from build123d import *

# Parameters (mm, degrees)
F0_R     = 2.25
F1_DEPTH = 0.2
F2_DEPTH = 1.2


with BuildPart() as f1:
    # F0 (on Top) → F1 (new body)
    with BuildSketch(Plane.XY):
        with BuildLine():
            Line((0.7, -5.554778), (0.7, -4.445222))
            ThreePointArc((0.7, -4.445222), (0, -4.5), (-0.7, -4.445222))
            Line((-0.7, -4.445222), (-0.7, -5.554778))
            ThreePointArc((-0.7, -5.554778), (0, -5.5), (0.7, -5.554778))
        make_face()
        with BuildLine():
            ThreePointArc((4.445222, 0.7), (4.486285, 0.35107), (4.5, 0))
            ThreePointArc((4.5, 0), (4.486285, -0.35107), (4.445222, -0.7))
            Line((4.445222, -0.7), (5.554778, -0.7))
            ThreePointArc((5.554778, -0.7), (5.5, 0), (5.554778, 0.7))
            Line((5.554778, 0.7), (4.445222, 0.7))
        make_face()
        with BuildLine():
            Line((5.554778, -9.3), (4.445222, -9.3))
            ThreePointArc((4.445222, -9.3), (4.486285, -9.64893), (4.5, -10))
            ThreePointArc((4.5, -10), (4.486285, -10.35107), (4.445222, -10.7))
            Line((4.445222, -10.7), (5.554778, -10.7))
            ThreePointArc((5.554778, -10.7), (5.5, -10), (5.554778, -9.3))
        make_face()
        with BuildLine():
            Line((15.554778, 0.7), (14.445222, 0.7))
            ThreePointArc((14.445222, 0.7), (14.486285, 0.35107), (14.5, 0))
            ThreePointArc((14.5, 0), (14.486285, -0.35107), (14.445222, -0.7))
            Line((14.445222, -0.7), (15.554778, -0.7))
            ThreePointArc((15.554778, -0.7), (15.5, 0), (15.554778, 0.7))
        make_face()
        with BuildLine():
            Line((15.554778, -9.3), (14.445222, -9.3))
            ThreePointArc((14.445222, -9.3), (14.486285, -9.64893), (14.5, -10))
            ThreePointArc((14.5, -10), (14.486285, -10.35107), (14.445222, -10.7))
            Line((14.445222, -10.7), (15.554778, -10.7))
            ThreePointArc((15.554778, -10.7), (15.5, -10), (15.554778, -9.3))
        make_face()
        with BuildLine():
            ThreePointArc((20.7, -4.445222), (20, -4.5), (19.3, -4.445222))
            Line((19.3, -4.445222), (19.3, -5.554778))
            ThreePointArc((19.3, -5.554778), (20, -5.5), (20.7, -5.554778))
            Line((20.7, -5.554778), (20.7, -4.445222))
        make_face()
        with BuildLine():
            ThreePointArc((4.445222, -9.3), (3.181981, -6.818019), (0.7, -5.554778))
            ThreePointArc((0.7, -5.554778), (0, -5.5), (-0.7, -5.554778))
            ThreePointArc((-0.7, -5.554778), (-4.5, -10), (-0.7, -14.445222))
            ThreePointArc((-0.7, -14.445222), (0, -14.5), (0.7, -14.445222))
            ThreePointArc((0.7, -14.445222), (3.181981, -13.181981), (4.445222, -10.7))
            ThreePointArc((4.445222, -10.7), (4.486285, -10.35107), (4.5, -10))
            ThreePointArc((4.5, -10), (4.486285, -9.64893), (4.445222, -9.3))
        make_face()
        with Locations((0, -10)):
            Circle(F0_R, mode=Mode.SUBTRACT)
        with BuildLine():
            ThreePointArc((24.445222, 0.7), (20, 4.5), (15.554778, 0.7))
            ThreePointArc((15.554778, 0.7), (15.5, 0), (15.554778, -0.7))
            ThreePointArc((15.554778, -0.7), (16.818019, -3.181981), (19.3, -4.445222))
            ThreePointArc((19.3, -4.445222), (20, -4.5), (20.7, -4.445222))
            ThreePointArc((20.7, -4.445222), (23.181981, -3.181981), (24.445222, -0.7))
            ThreePointArc((24.445222, -0.7), (24.486285, -0.35107), (24.5, 0))
            ThreePointArc((24.5, 0), (24.486285, 0.35107), (24.445222, 0.7))
        make_face()
        with Locations((20, 0)):
            Circle(F0_R, mode=Mode.SUBTRACT)
        with BuildLine():
            ThreePointArc((20.7, -5.554778), (20, -5.5), (19.3, -5.554778))
            ThreePointArc((19.3, -5.554778), (16.818019, -6.818019), (15.554778, -9.3))
            ThreePointArc((15.554778, -9.3), (15.5, -10), (15.554778, -10.7))
            ThreePointArc((15.554778, -10.7), (16.818019, -13.181981), (19.3, -14.445222))
            ThreePointArc((19.3, -14.445222), (20, -14.5), (20.7, -14.445222))
            ThreePointArc((20.7, -14.445222), (23.181981, -13.181981), (24.445222, -10.7))
            ThreePointArc((24.445222, -10.7), (24.486285, -10.35107), (24.5, -10))
            ThreePointArc((24.5, -10), (24.486285, -9.64893), (24.445222, -9.3))
            ThreePointArc((24.445222, -9.3), (23.181981, -6.818019), (20.7, -5.554778))
        make_face()
        with Locations((20, -10)):
            Circle(F0_R, mode=Mode.SUBTRACT)
        with BuildLine():
            ThreePointArc((14.445222, 0.7), (10, 4.5), (5.554778, 0.7))
            ThreePointArc((5.554778, 0.7), (5.5, 0), (5.554778, -0.7))
            ThreePointArc((5.554778, -0.7), (6.818019, -3.181981), (9.3, -4.445222))
            ThreePointArc((9.3, -4.445222), (10, -4.5), (10.7, -4.445222))
            ThreePointArc((10.7, -4.445222), (13.181981, -3.181981), (14.445222, -0.7))
            ThreePointArc((14.445222, -0.7), (14.486285, -0.35107), (14.5, 0))
            ThreePointArc((14.5, 0), (14.486285, 0.35107), (14.445222, 0.7))
        make_face()
        with Locations((10, 0)):
            Circle(F0_R, mode=Mode.SUBTRACT)
        with BuildLine():
            ThreePointArc((10.7, -5.554778), (10, -5.5), (9.3, -5.554778))
            ThreePointArc((9.3, -5.554778), (6.818019, -6.818019), (5.554778, -9.3))
            ThreePointArc((5.554778, -9.3), (5.5, -10), (5.554778, -10.7))
            ThreePointArc((5.554778, -10.7), (6.818019, -13.181981), (9.3, -14.445222))
            ThreePointArc((9.3, -14.445222), (10, -14.5), (10.7, -14.445222))
            ThreePointArc((10.7, -14.445222), (13.181981, -13.181981), (14.445222, -10.7))
            ThreePointArc((14.445222, -10.7), (14.486285, -10.35107), (14.5, -10))
            ThreePointArc((14.5, -10), (14.486285, -9.64893), (14.445222, -9.3))
            ThreePointArc((14.445222, -9.3), (13.181981, -6.818019), (10.7, -5.554778))
        make_face()
        with Locations((10, -10)):
            Circle(F0_R, mode=Mode.SUBTRACT)
        with BuildLine():
            ThreePointArc((4.445222, -0.7), (4.486285, -0.35107), (4.5, 0))
            ThreePointArc((4.5, 0), (4.486285, 0.35107), (4.445222, 0.7))
            ThreePointArc((4.445222, 0.7), (0, 4.5), (-4.445222, 0.7))
            ThreePointArc((-4.445222, 0.7), (-4.5, 0), (-4.445222, -0.7))
            ThreePointArc((-4.445222, -0.7), (-3.181981, -3.181981), (-0.7, -4.445222))
            ThreePointArc((-0.7, -4.445222), (0, -4.5), (0.7, -4.445222))
            ThreePointArc((0.7, -4.445222), (3.181981, -3.181981), (4.445222, -0.7))
        make_face()
        Circle(F0_R, mode=Mode.SUBTRACT)
        with BuildLine():
            ThreePointArc((10.7, -4.445222), (10, -4.5), (9.3, -4.445222))
            Line((9.3, -4.445222), (9.3, -5.554778))
            ThreePointArc((9.3, -5.554778), (10, -5.5), (10.7, -5.554778))
            Line((10.7, -5.554778), (10.7, -4.445222))
        make_face()
    extrude(amount=-F1_DEPTH)

    # F0 (on Top) → F2 (join)
    with BuildSketch(Plane.XY):
        with BuildLine():
            ThreePointArc((4.445222, -0.7), (4.486285, -0.35107), (4.5, 0))
            ThreePointArc((4.5, 0), (4.486285, 0.35107), (4.445222, 0.7))
            ThreePointArc((4.445222, 0.7), (0, 4.5), (-4.445222, 0.7))
            ThreePointArc((-4.445222, 0.7), (-4.5, 0), (-4.445222, -0.7))
            ThreePointArc((-4.445222, -0.7), (-3.181981, -3.181981), (-0.7, -4.445222))
            ThreePointArc((-0.7, -4.445222), (0, -4.5), (0.7, -4.445222))
            ThreePointArc((0.7, -4.445222), (3.181981, -3.181981), (4.445222, -0.7))
        make_face()
        Circle(F0_R, mode=Mode.SUBTRACT)
        with BuildLine():
            ThreePointArc((14.445222, 0.7), (10, 4.5), (5.554778, 0.7))
            ThreePointArc((5.554778, 0.7), (5.5, 0), (5.554778, -0.7))
            ThreePointArc((5.554778, -0.7), (6.818019, -3.181981), (9.3, -4.445222))
            ThreePointArc((9.3, -4.445222), (10, -4.5), (10.7, -4.445222))
            ThreePointArc((10.7, -4.445222), (13.181981, -3.181981), (14.445222, -0.7))
            ThreePointArc((14.445222, -0.7), (14.486285, -0.35107), (14.5, 0))
            ThreePointArc((14.5, 0), (14.486285, 0.35107), (14.445222, 0.7))
        make_face()
        with Locations((10, 0)):
            Circle(F0_R, mode=Mode.SUBTRACT)
        with BuildLine():
            ThreePointArc((24.445222, 0.7), (20, 4.5), (15.554778, 0.7))
            ThreePointArc((15.554778, 0.7), (15.5, 0), (15.554778, -0.7))
            ThreePointArc((15.554778, -0.7), (16.818019, -3.181981), (19.3, -4.445222))
            ThreePointArc((19.3, -4.445222), (20, -4.5), (20.7, -4.445222))
            ThreePointArc((20.7, -4.445222), (23.181981, -3.181981), (24.445222, -0.7))
            ThreePointArc((24.445222, -0.7), (24.486285, -0.35107), (24.5, 0))
            ThreePointArc((24.5, 0), (24.486285, 0.35107), (24.445222, 0.7))
        make_face()
        with Locations((20, 0)):
            Circle(F0_R, mode=Mode.SUBTRACT)
        with BuildLine():
            ThreePointArc((20.7, -5.554778), (20, -5.5), (19.3, -5.554778))
            ThreePointArc((19.3, -5.554778), (16.818019, -6.818019), (15.554778, -9.3))
            ThreePointArc((15.554778, -9.3), (15.5, -10), (15.554778, -10.7))
            ThreePointArc((15.554778, -10.7), (16.818019, -13.181981), (19.3, -14.445222))
            ThreePointArc((19.3, -14.445222), (20, -14.5), (20.7, -14.445222))
            ThreePointArc((20.7, -14.445222), (23.181981, -13.181981), (24.445222, -10.7))
            ThreePointArc((24.445222, -10.7), (24.486285, -10.35107), (24.5, -10))
            ThreePointArc((24.5, -10), (24.486285, -9.64893), (24.445222, -9.3))
            ThreePointArc((24.445222, -9.3), (23.181981, -6.818019), (20.7, -5.554778))
        make_face()
        with Locations((20, -10)):
            Circle(F0_R, mode=Mode.SUBTRACT)
        with BuildLine():
            ThreePointArc((10.7, -5.554778), (10, -5.5), (9.3, -5.554778))
            ThreePointArc((9.3, -5.554778), (6.818019, -6.818019), (5.554778, -9.3))
            ThreePointArc((5.554778, -9.3), (5.5, -10), (5.554778, -10.7))
            ThreePointArc((5.554778, -10.7), (6.818019, -13.181981), (9.3, -14.445222))
            ThreePointArc((9.3, -14.445222), (10, -14.5), (10.7, -14.445222))
            ThreePointArc((10.7, -14.445222), (13.181981, -13.181981), (14.445222, -10.7))
            ThreePointArc((14.445222, -10.7), (14.486285, -10.35107), (14.5, -10))
            ThreePointArc((14.5, -10), (14.486285, -9.64893), (14.445222, -9.3))
            ThreePointArc((14.445222, -9.3), (13.181981, -6.818019), (10.7, -5.554778))
        make_face()
        with Locations((10, -10)):
            Circle(F0_R, mode=Mode.SUBTRACT)
        with BuildLine():
            ThreePointArc((4.445222, -9.3), (3.181981, -6.818019), (0.7, -5.554778))
            ThreePointArc((0.7, -5.554778), (0, -5.5), (-0.7, -5.554778))
            ThreePointArc((-0.7, -5.554778), (-4.5, -10), (-0.7, -14.445222))
            ThreePointArc((-0.7, -14.445222), (0, -14.5), (0.7, -14.445222))
            ThreePointArc((0.7, -14.445222), (3.181981, -13.181981), (4.445222, -10.7))
            ThreePointArc((4.445222, -10.7), (4.486285, -10.35107), (4.5, -10))
            ThreePointArc((4.5, -10), (4.486285, -9.64893), (4.445222, -9.3))
        make_face()
        with Locations((0, -10)):
            Circle(F0_R, mode=Mode.SUBTRACT)
    extrude(amount=F2_DEPTH)


solid = f1.part
Input: part model. Units: mm. Frame: model coordinates. Give positions to 0.01 mm unless a question says otherwise; leave off trailing zeros. Order: outer loops, then holes, each group sorted by start corner. A loop starts at its lowest first (then second) coordinate and runs counter-clockwise, first axis right, second up. Notation, with made-up numbers: (-25.75, 86.5) - (9.25, 86.5) arc R35 cw to (9.25, 125.5) - close; hole circle Ø6 at (7.5, 58.5). An arc over 180 degrees is marked (long way). Answer as a JSON object with one key per item and string values. Group by question number.
Q1. Cut plane A-A, the plane x = 20. Output: boundary loops of the cut face in (y, z), then the cut area to 3 significant figures.
Q2. Line query: probe 1 along Y at (x, z) = (0, 0.35); probe 2 along X at (y, z) = (-10.25, 0.55); probe 3 along Y at (x, z) = (0, -0.05). Output: solid intervals per line, ascending.
Q3. Cut plane D-D, the plane y = -9. Output: boundary loops of the cut face in (x, z).
Q4. First-contact query: pin 1 Ø4 at (x, y) = (20, 0) entering from +Z; pin 2 Ø0.9 at (x, y) = (20, -5) entering from +Z. Flat tips, straight axial feed; report the tip coordinate or a pass-through.
Q5. Cut plane B-B, the plane z = 0.8. Count the separate pieces of the cut face and the enclosed holes in it, then the cut area to 3 significant figures.
Q6. Mould query, pull axis X, two halves, no side actions, for faces 1 (the face through (-4.5, -9.9, 0.5)), 2 (the face through (10.1, 4.5, 0.5)), 3 (the face through (2, -2, 1.2)). Classes: pulls with the +X half, pulls with the -X half, needs draft (parallel to the pull), parting line crosses it, or undercut.
Q7. Cut plane C-C, the plane y = -6.5. Output: boundary loops of the cut face in (x, z), then the cut area to 3 significant figures.
Results:
{
 "1": {"outline": "(-14.5, -0.2) - (-12.25, -0.2) - (-12.25, 1.2) - (-14.5, 1.2) - close; (-7.75, -0.2) - (-2.25, -0.2) - (-2.25, 1.2) - (-4.5, 1.2) - (-4.5, 0) - (-5.5, 0) - (-5.5, 1.2) - (-7.75, 1.2) - close; (2.25, -0.2) - (4.5, -0.2) - (4.5, 1.2) - (2.25, 1.2) - close", "area": "12.8 mm^2"},
 "2": {"probe 1": "-14.5 to -12.25, -7.75 to -5.5, -4.5 to -2.25, 2.25 to 4.5", "probe 2": "-4.49 to -2.24, 2.24 to 4.49, 5.51 to 7.76, 12.24 to 14.49, 15.51 to 17.76, 22.24 to 24.49", "probe 3": "-14.5 to -12.25, -7.75 to -2.25, 2.25 to 4.5"},
 "3": {"outline": "(-4.39, -0.2) - (-2.02, -0.2) - (-2.02, 1.2) - (-4.39, 1.2) - close; (2.02, -0.2) - (4.39, -0.2) - (4.39, 1.2) - (2.02, 1.2) - close; (5.61, -0.2) - (7.98, -0.2) - (7.98, 1.2) - (5.61, 1.2) - close; (12.02, -0.2) - (14.39, -0.2) - (14.39, 1.2) - (12.02, 1.2) - close; (15.61, -0.2) - (17.98, -0.2) - (17.98, 1.2) - (15.61, 1.2) - close; (22.02, -0.2) - (24.39, -0.2) - (24.39, 1.2) - (22.02, 1.2) - close"},
 "4": {"pin 1": "through", "pin 2": "z = 0"},
 "5": {"separate pieces": "6", "enclosed holes": "6", "area": "286 mm^2"},
 "6": {"face 1": "pulls with the -X half", "face 2": "undercut", "face 3": "needs draft"},
 "7": {"outline": "(-2.83, -0.2) - (2.83, -0.2) - (2.83, 1.2) - (-2.83, 1.2) - close; (7.17, -0.2) - (12.83, -0.2) - (12.83, 1.2) - (7.17, 1.2) - close; (17.17, -0.2) - (22.83, -0.2) - (22.83, 1.2) - (17.17, 1.2) - close", "area": "23.8 mm^2"}
}
